Can you work these out from the model? Positions are in its coordinate system, mm. A direction names the side the tool comes from. Coordinates: 2 decimals unless noted, no trailing zeros. Order: outer loops, then holes, each group sorted by start corner. A loop starts at its lowest first (then second) coordinate and runs counter-clockwise, first axis right, second up. Notation, with made-up numbers: (-5.75, 31) -> (29.25, 31) arc R18 ccw to (29.25, 61) -> close; hole circle Ø5 at (80.5, -12). An arc over 180 degrees is marked (long way). Answer as CSV lines item,"result".
from build123d import *

# Parameters (mm, degrees)
SKETCH1_W           = 100
SKETCH1_H           = 24
SKETCH1_R           = 3.5
BOSS_EXTRUDE1_DEPTH = 5
BOSS_EXTRUDE2_DEPTH = 9
SKETCH3_R           = 8
CUT_EXTRUDE1_DEPTH  = 4


with BuildPart() as part:
    # Sketch1 → Boss-Extrude1 (new body)
    with BuildSketch(Plane(origin=(0, 0, 0), x_dir=(1, 0, 0), z_dir=(0, 1, 0))):
        Rectangle(SKETCH1_W, SKETCH1_H)
        with Locations((-45, 7)):
            Circle(SKETCH1_R, mode=Mode.SUBTRACT)
        with Locations((-45, -7)):
            Circle(SKETCH1_R, mode=Mode.SUBTRACT)
        with Locations((45, 7)):
            Circle(SKETCH1_R, mode=Mode.SUBTRACT)
        with Locations((45, -7)):
            Circle(SKETCH1_R, mode=Mode.SUBTRACT)
    extrude(amount=BOSS_EXTRUDE1_DEPTH)

    # Sketch2 → Boss-Extrude2 (add)
    with BuildSketch(Plane.XY.offset(3)):
        with BuildLine():
            Line((-29.978021695, 5), (29.763516014, 5))
            Line((29.763516014, 5), (11.035619534, 51.854874594))
            ThreePointArc((11.035619534, 51.854874594), (-0.107252841, 59.401067767), (-11.250125215, 51.854874594))
            Line((-11.250125215, 51.854874594), (-29.978021695, 5))
        make_face()
    extrude(amount=BOSS_EXTRUDE2_DEPTH)

    # Sketch3 → Cut-Extrude1 (cut)
    with BuildSketch(Plane(origin=(0, 0, 3), x_dir=(-1, 0, 0), z_dir=(0, 0, -1))):
        with Locations((0, 49.578279074)):
            Circle(SKETCH3_R)
    extrude(amount=-CUT_EXTRUDE1_DEPTH, mode=Mode.SUBTRACT)


solid = part.part
Q1. We'd pull the mould along Z, two halves only. Please class faces 3 (the flat face through (-1, 23, 12)), 4 (the flat face through (-1, 27, 3)), 5 (the cylindrical face through (1.04, 57.51, 4.97)), 6 (the cylindrical face through (-48.497, 2.465, -7.154)): pulls with the +Z half, pulls with the -Z half, needs draft (parallel to the pull), parting line crosses it, or undercut.
Solution:
face 3,"pulls with the +Z half"
face 4,"pulls with the -Z half"
face 5,"needs draft"
face 6,"undercut"
Q2. Imagine slicing it at C-C (x = 0). List the corners of the cut face in (y, z) for me, and give its area (3 significant figures).
Solution:
outline,"(0, -12) -> (5, -12) -> (5, 3) -> (41.58, 3) -> (41.58, 7) -> (57.58, 7) -> (57.58, 3) -> (59.4, 3) -> (59.4, 12) -> (0, 12) -> close"
area,"546 mm2"
Q3. Imagine slicing it at B-B (x = -45). List the corners of the cut face in (y, z) for me, and give its area (3 significant figures).
Solution:
outline,"(0, -12) -> (5, -12) -> (5, -10.5) -> (0, -10.5) -> close; (0, -3.5) -> (5, -3.5) -> (5, 3.5) -> (0, 3.5) -> close; (0, 10.5) -> (5, 10.5) -> (5, 12) -> (0, 12) -> close"
area,"50.0 mm2"
Q4. Which directions (+Z, -Z, +X, -X, +Y, -Y) give clear straight access to the entire face, cutting with the end or side of a thin tool? Please do faces 1 (the flat face through (0, 50, 7)), 2 (the cylindrical face through (41.503, 2.465, -7.154)).
Solution:
face 1,"-Z"
face 2,"+Y, -Y"
Q5. Imagine slicing it at A-A (z = -7). List the corners of the cut face in (x, y) for me.
Solution:
outline,"(-50, 0) -> (-48.5, 0) -> (-48.5, 5) -> (-50, 5) -> close; (-41.5, 0) -> (41.5, 0) -> (41.5, 5) -> (-41.5, 5) -> close; (48.5, 0) -> (50, 0) -> (50, 5) -> (48.5, 5) -> close"
Q6. For P1, Ø8, axis at x = -13, y = 25, coming from the -Z side; P2, Ø8, axis at x = -21, y = 41.5, coming from the -Z side; P3, Ø3, axis at y = 19, z = 5, coming from the +X side; P4, Ø11, axis at x = 45, z = -7, coming from the +Y side, each with a flat end and sliding along its axis, tell me the tip position at first contact or that it passes through.
Solution:
P1,"z = 3"
P2,"through"
P3,"x = 24.77"
P4,"y = 5"
Q7. If I drill on line 1 (X direction, y = 1, z = -7); line 2 (Z direction, x = -45, y = 1.5); line 3 (Y direction, x = 0, z = 4.4), over which ranges is the centre line in solid material (lowest first)?
Solution:
line 1,"-50 to -48.5, -41.5 to 41.5, 48.5 to 50"
line 2,"-12 to -10.5, -3.5 to 3.5, 10.5 to 12"
line 3,"0 to 41.58, 57.58 to 59.4"
Q8. Imagine slicing it at D-D (z = -0.5). List the corners of the cut face in (x, y) for me, and give its area (3 significant figures).
Solution:
outline,"(-50, 0) -> (50, 0) -> (50, 5) -> (-50, 5) -> close"
area,"500 mm2"
